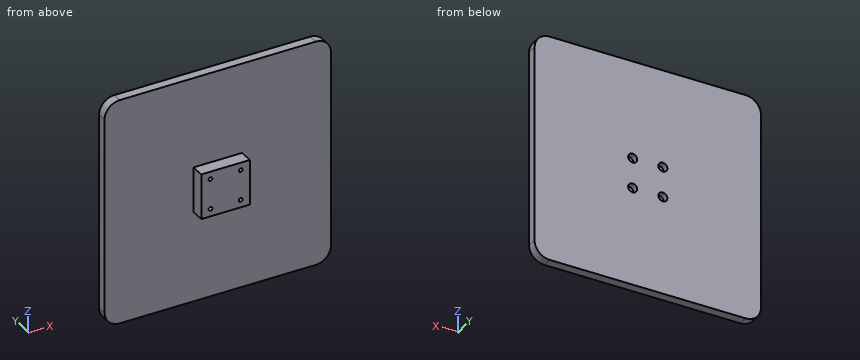
from build123d import *

# Parameters (mm, degrees)
SKETCH2_W           = 150
SKETCH2_H           = 150
SKETCH2_R           = 1.25
BOSS_EXTRUDE1_DEPTH = 6.35
FILLET1_R           = 10
SKETCH3_R           = 3
CUT_EXTRUDE1_DEPTH  = 4.3
BOSS_EXTRUDE2_START = 9
SKETCH4_W           = 32.2
SKETCH4_H           = 30
SKETCH4_R           = 1.25
BOSS_EXTRUDE2_DEPTH = 9


with BuildPart() as part:
    # Sketch2 → Boss-Extrude1 (new body)
    with BuildSketch(Plane(origin=(0, 0, 0), x_dir=(1, 0, 0), z_dir=(0, 1, 0))):
        with Locations((-75, 75)):
            Rectangle(SKETCH2_W, SKETCH2_H)
        with Locations(Location((-85, 85, 0), (0, 0, 270))):
            Circle(SKETCH2_R, mode=Mode.SUBTRACT)
        with Locations(Location((-65, 85, 0), (0, 0, 270))):
            Circle(SKETCH2_R, mode=Mode.SUBTRACT)
        with Locations(Location((-85, 65, 0), (0, 0, 270))):
            Circle(SKETCH2_R, mode=Mode.SUBTRACT)
        with Locations(Location((-65, 65, 0), (0, 0, 270))):
            Circle(SKETCH2_R, mode=Mode.SUBTRACT)
    extrude(amount=BOSS_EXTRUDE1_DEPTH)

    # Fillet1
    fillet1_edges = [part.edges().sort_by_distance(p)[0] for p in [
        (0, 3.175, 0),
        (-150, 3.175, 0),
        (-150, 3.175, -150),
        (0, 3.175, -150),
    ]]
    fillet(fillet1_edges, radius=FILLET1_R)

    # Sketch3 → Cut-Extrude1 (cut)
    with BuildSketch(Plane(origin=(0, 6.35, 0), x_dir=(1, 0, 0), z_dir=(0, 1, 0))):
        with Locations(Location((-85, 85, 0), (0, 0, 270))):
            Circle(SKETCH3_R)
        with Locations(Location((-65, 85, 0), (0, 0, 270))):
            Circle(SKETCH3_R)
        with Locations(Location((-85, 65, 0), (0, 0, 270))):
            Circle(SKETCH3_R)
        with Locations(Location((-65, 65, 0), (0, 0, 270))):
            Circle(SKETCH3_R)
    extrude(amount=-CUT_EXTRUDE1_DEPTH, mode=Mode.SUBTRACT)

    # Sketch4 → Boss-Extrude2 (add)
    with BuildSketch(Plane.XZ.offset(BOSS_EXTRUDE2_START)):
        with Locations((-75, -75)):
            Rectangle(SKETCH4_W, SKETCH4_H)
        with Locations(Location((-85, -65, 0), (0, 0, 270))):
            Circle(SKETCH4_R, mode=Mode.SUBTRACT)
        with Locations(Location((-85, -85, 0), (0, 0, 270))):
            Circle(SKETCH4_R, mode=Mode.SUBTRACT)
        with Locations(Location((-65, -85, 0), (0, 0, 270))):
            Circle(SKETCH4_R, mode=Mode.SUBTRACT)
        with Locations(Location((-65, -65, 0), (0, 0, 270))):
            Circle(SKETCH4_R, mode=Mode.SUBTRACT)
    extrude(amount=-BOSS_EXTRUDE2_DEPTH)


solid = part.part
Work out the finished part from the listing and answer in its coordinate system (mm). Give positions to 0.01 mm unless a question says otherwise; leave off trailing zeros. Loops run counter-clockwise (first coordinate to the right, second up) from the corner with the lowest first, then second, coordinate; pieces in that order, holes last. Notation, with made-up numbers: (-38.5, 83) - (-14.5, 83) arc R5 ccw to (-14.5, 87) - close; hole circle Ø8 at (12, -5). An arc over 180 degrees is marked (long way). Answer in a Markdown table with one row per item. Add a question column.
Q1. The part is cut by section D-D (x = -47). Determine the outline of the cut face in (y, z), and give its area (4 significant figures).
Q2. Each of these flat-tipped pins is pushed along its axis until it touches: P1, Ø4.5, axis at x = -78.5, y = -6, coming from the +Z side; P2, Ø2.5, axis at y = -5.5, z = -69, coming from the -X side; P3, Ø2.5, axis at y = -6, z = -81.5, coming from the +X side. Where does it stop, or does it pass through?
Q3. The part is cut by section C-C (z = -27.5). Determine the outline of the cut face in (x, y), and give its area (4 significant figures).
Q4. Consider line 1 along Z through (x, y) = (-65, 1.3); line 2 along Z through (x, y) = (-65, -3). Determine where each line is inside the solid, lowest interval first.
Q5. The part is cut by section A-A (x = -77). Determine the outline of the cut face in (y, z), and give its area (3 significant figures).
Solution:
| question | item | result |
|---|---|---|
| 1 | outline | (0, -150) - (6.35, -150) - (6.35, 0) - (0, 0) - close |
| 1 | area | 952.5 mm² |
| 2 | P1 | stops at z = -60 |
| 2 | P2 | stops at x = -91.1 |
| 2 | P3 | stops at x = -58.9 |
| 3 | outline | (-150, 0) - (0, 0) - (0, 6.35) - (-150, 6.35) - close |
| 3 | area | 952.5 mm² |
| 4 | line 1 | z = -150 to -86.25, -83.75 to -66.25, -63.75 to 0 |
| 4 | line 2 | z = -90 to -86.25, -83.75 to -66.25, -63.75 to -60 |
| 5 | outline | (-9, -90) - (0, -90) - (0, -150) - (6.35, -150) - (6.35, 0) - (0, 0) - (0, -60) - (-9, -60) - close |
| 5 | area | 1,220 mm² |
